Read the model definition and answer for the solid it produces. Units are mm, in the model's axes. Coordinates: 2 decimals unless noted, no trailing zeros. Write each loop counter-clockwise with the first axis right and the second up, starting at its lowest first coordinate (ties: lowest second). Pieces come first, ordered by that corner, then holes.
(1) Find the intervals of material crossed by probe 1 along Y at (x, z) = (-105, 1.3); probe 2 along X at (y, z) = (-54, 3.2); probe 3 along X at (y, z) = (-92.5, 1.35), in increasing order.
(2) Section B-B on y = -23.5 is taken. Write down the section's boundary in (x, z), then the cut area to 3 significant figures.
(3) Given pin 1 (3 mm diameter, centred on x = -37.66, y = -52.74, fed in from -Z), flat-ended and moving along its own axis, determine where the tip first touches the part or whether it passes through.
(4) Section A-A on y = 76 is taken. Write down the section's boundary in (x, z).
from build123d import *

# Parameters (mm, degrees)
SKETCH1_W               = 250
SKETCH1_H               = 275
BOSS_EXTRUDE1_DEPTH     = 4.2
ESQUISSE1_R             = 2.50000008
ENL_V_MAT_EXTRU_1_DEPTH = 5.2


with BuildPart() as part:
    # Sketch1 → Boss-Extrude1 (new body)
    with BuildSketch(Plane.XY):
        with Locations((-95.228215768, -27.385892116)):
            Rectangle(SKETCH1_W, SKETCH1_H)
    extrude(amount=BOSS_EXTRUDE1_DEPTH)

    # Esquisse1 → Enlèv. mat.-Extru.1 (cut, through all)
    with BuildSketch(Plane.XY.offset(4.2)):
        with Locations((-37.655669773, -94.649179191)):
            Circle(ESQUISSE1_R)
        with Locations((-37.655669773, -52.739179191)):
            Circle(ESQUISSE1_R)
        with Locations((-109.410669773, -94.649179191)):
            Circle(ESQUISSE1_R)
        with Locations((-109.410669773, -52.739179191)):
            Circle(ESQUISSE1_R)
        with BuildLine():
            Line((-110.228215768, 70.114107884), (-80.228215768, 70.114107884))
            ThreePointArc((-80.228215768, 70.114107884), (-95.228215768, 85.114107884), (-110.228215768, 70.114107884))
        make_face()
        with BuildLine():
            Line((-111.073893882, -15.305892116), (-79.382537653, -15.305892116))
            ThreePointArc((-79.382537653, -15.305892116), (-95.228215768, -31.151570231), (-111.073893882, -15.305892116))
        make_face()
    extrude(amount=-ENL_V_MAT_EXTRU_1_DEPTH, mode=Mode.SUBTRACT)


solid = part.part
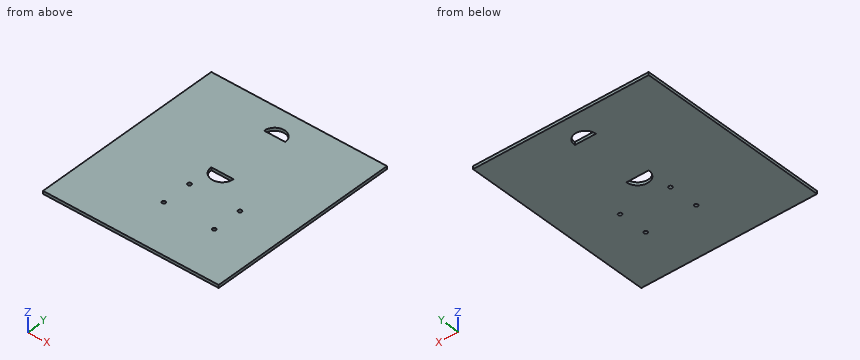
Response:
1. probe 1: y = -164.89 to -27.78, -15.31 to 70.11, 81.49 to 110.11
1. probe 2: x = -220.23 to -111.57, -107.25 to -39.81, -35.5 to 29.77
1. probe 3: x = -220.23 to -110.69, -108.13 to -38.93, -36.38 to 29.77
2. outline: (-220.23, 0) - (-108.79, 0) - (-108.79, 4.2) - (-220.23, 4.2) - close; (-81.67, 0) - (29.77, 0) - (29.77, 4.2) - (-81.67, 4.2) - close
2. area: 936 mm2
3. pin 1: passes through
4. outline: (-220.23, 0) - (-109.03, 0) - (-109.03, 4.2) - (-220.23, 4.2) - close; (-81.43, 0) - (29.77, 0) - (29.77, 4.2) - (-81.43, 4.2) - close
